```python
from build123d import *

# Parameters (mm, degrees)
BOSS_EXTRUDE1_DEPTH = 30
SKETCH2_R           = 2.25
CUT_EXTRUDE1_DEPTH  = 15
FILLET1_R           = 5
CHAMFER1_SIZE       = 20
CHAMFER1_SIZE_2     = 54.949548389
SKETCH3_W           = 25
SKETCH3_H           = 39.596952294
CUT_EXTRUDE2_DEPTH  = 15
SKETCH4_R           = 1.75
CUT_EXTRUDE3_DEPTH  = 65.75337829
CHAMFER2_SIZE       = 1
SKETCH5_R           = 2
CUT_EXTRUDE4_DEPTH  = 56.767373974
SKETCH6_R           = 7.5
CUT_EXTRUDE5_DEPTH  = 25
FILLET2_R           = 2
FILLET3_R           = 5


with BuildPart() as part:
    # Sketch1 → Boss-Extrude1 (new body)
    with BuildSketch(Plane.XY):
        with BuildLine():
            Line((-12, 0), (-12, -30))
            Line((-12, -30), (-19, -30))
            Line((-19, -30), (-19, 43))
            Line((-19, 43), (19, 43))
            Line((19, 43), (19, -30))
            Line((19, -30), (12, -30))
            Line((12, -30), (12, 0))
            ThreePointArc((12, 0), (0, 12), (-12, 0))
        make_face()
    extrude(amount=BOSS_EXTRUDE1_DEPTH)

    # Sketch2 → Cut-Extrude1 (cut)
    with BuildSketch(Plane.XZ.offset(30)):
        with Locations(Location((-15, 5, 0), (0, 0, 270))):
            Circle(SKETCH2_R)
        with Locations(Location((15, 5, 0), (0, 0, 270))):
            Circle(SKETCH2_R)
        with Locations(Location((-15, 15, 0), (0, 0, 270))):
            Circle(SKETCH2_R)
        with Locations(Location((15, 15, 0), (0, 0, 270))):
            Circle(SKETCH2_R)
        with Locations(Location((-15, 25, 0), (0, 0, 270))):
            Circle(SKETCH2_R)
        with Locations(Location((15, 25, 0), (0, 0, 270))):
            Circle(SKETCH2_R)
    extrude(amount=-CUT_EXTRUDE1_DEPTH, mode=Mode.SUBTRACT)

    # Fillet1
    fillet1_edges = [part.edges().sort_by_distance(p)[0] for p in [
        (0, 43, 0),
    ]]
    fillet(fillet1_edges, radius=FILLET1_R)

    # Chamfer1
    # the kernel refuses this chamfer: 54.949548389, 20 mm, written as the material it takes off along each edge
    with BuildSketch(Plane(origin=(-161.549828987, 43, 30), x_dir=(0, 0.09904090225205052, -0.9950833631817486), z_dir=(1, 0, 0))) as chamfer1_piece_1:
        Polygon((CHAMFER1_SIZE * 0.995083363182, -CHAMFER1_SIZE * 0.0990409022521), (-CHAMFER1_SIZE_2 * 0.0990409022522, -CHAMFER1_SIZE_2 * 0.995083363183), (0, 0), align=None)
    extrude(amount=323.099657974, mode=Mode.SUBTRACT)

    # Sketch3 → Cut-Extrude2 (cut)
    with BuildSketch(Plane(origin=(0, 43, 0), x_dir=(1, 0, 0), z_dir=(0, 1, 0))):
        Rectangle(SKETCH3_W, SKETCH3_H)
    extrude(amount=-CUT_EXTRUDE2_DEPTH, mode=Mode.SUBTRACT)

    # Sketch4 → Cut-Extrude3 (cut, through all)
    with BuildSketch(Plane.ZY.offset(19)):
        with Locations((5, 38)):
            Circle(SKETCH4_R)
    extrude(amount=-CUT_EXTRUDE3_DEPTH, mode=Mode.SUBTRACT)

    # Chamfer2
    # the kernel refuses this chamfer: 1 mm, written as the material it takes off along each edge
    with BuildSketch(Plane(origin=(-15, -30, 25), x_dir=(0, 0, -1), z_dir=(-1, 0, 0))) as chamfer2_piece_1:
        Polygon((2.25 + CHAMFER2_SIZE, 0), (2.25, -CHAMFER2_SIZE), (2.25, 0), align=None)
    revolve(axis=Axis((-15, -30, 25), (0, -1, 0)), mode=Mode.SUBTRACT)
    with BuildSketch(Plane(origin=(15, -30, 15), x_dir=(0, 0, -1), z_dir=(-1, 0, 0))) as chamfer2_piece_2:
        Polygon((2.25 + CHAMFER2_SIZE, 0), (2.25, -CHAMFER2_SIZE), (2.25, 0), align=None)
    revolve(axis=Axis((15, -30, 15), (0, -1, 0)), mode=Mode.SUBTRACT)
    with BuildSketch(Plane(origin=(-15, -30, 15), x_dir=(0, 0, -1), z_dir=(-1, 0, 0))) as chamfer2_piece_3:
        Polygon((2.25 + CHAMFER2_SIZE, 0), (2.25, -CHAMFER2_SIZE), (2.25, 0), align=None)
    revolve(axis=Axis((-15, -30, 15), (0, -1, 0)), mode=Mode.SUBTRACT)
    with BuildSketch(Plane(origin=(15, -30, 5), x_dir=(0, 0, -1), z_dir=(-1, 0, 0))) as chamfer2_piece_4:
        Polygon((2.25 + CHAMFER2_SIZE, 0), (2.25, -CHAMFER2_SIZE), (2.25, 0), align=None)
    revolve(axis=Axis((15, -30, 5), (0, -1, 0)), mode=Mode.SUBTRACT)
    with BuildSketch(Plane(origin=(15, -30, 25), x_dir=(0, 0, -1), z_dir=(-1, 0, 0))) as chamfer2_piece_5:
        Polygon((2.25 + CHAMFER2_SIZE, 0), (2.25, -CHAMFER2_SIZE), (2.25, 0), align=None)
    revolve(axis=Axis((15, -30, 25), (0, -1, 0)), mode=Mode.SUBTRACT)
    with BuildSketch(Plane(origin=(-15, -30, 5), x_dir=(0, 0, -1), z_dir=(-1, 0, 0))) as chamfer2_piece_6:
        Polygon((2.25 + CHAMFER2_SIZE, 0), (2.25, -CHAMFER2_SIZE), (2.25, 0), align=None)
    revolve(axis=Axis((-15, -30, 5), (0, -1, 0)), mode=Mode.SUBTRACT)

    # Sketch5 → Cut-Extrude4 (cut, through all)
    with BuildSketch(Plane(origin=(0, 0, 0), x_dir=(-1, 0, 0), z_dir=(0, 0, -1))):
        with Locations((0, 23)):
            Circle(SKETCH5_R)
    extrude(amount=-CUT_EXTRUDE4_DEPTH, mode=Mode.SUBTRACT)

    # Sketch6 → Cut-Extrude5 (cut)
    with BuildSketch(Plane.XY.offset(30)):
        with Locations((0, 23)):
            Circle(SKETCH6_R)
    extrude(amount=-CUT_EXTRUDE5_DEPTH, mode=Mode.SUBTRACT)

    # Fillet2
    fillet2_edges = [part.edges().sort_by_distance(p)[0] for p in [
        (-5.590169944, 28, 10.229776757),
        (5.590169944, 28, 10.229776757),
    ]]
    fillet(fillet2_edges, radius=FILLET2_R)

    # Fillet3
    fillet3_edges = [part.edges().sort_by_distance(p)[0] for p in [
        (-15.75, 43, 10),
        (15.75, 43, 10),
    ]]
    fillet(fillet3_edges, radius=FILLET3_R)


solid = part.part
```
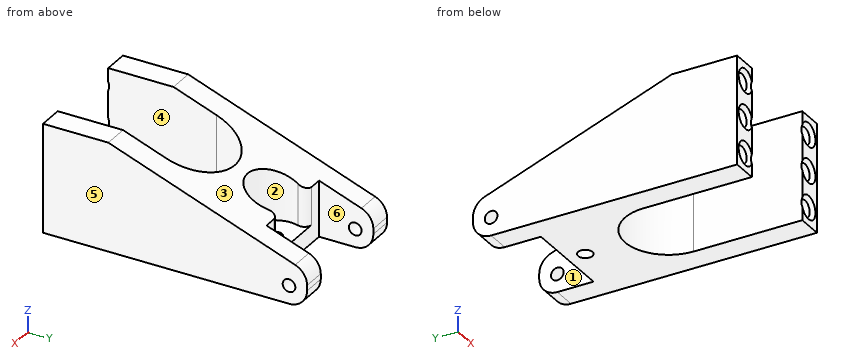
Check sheet for the modelled part. Datum: model origin and axes. Units: mm. Face numbers are marked on the shaded views. A direction names the side the tool comes from. Give positions to 0.01 mm unless a question says otherwise; leave off trailing zeros. Order: outer loops, then holes, each group sorted by start corner. A loop starts at its lowest first (then second) coordinate and runs counter-clockwise, first axis right, second up. Notation, with made-up numbers: M 7.25,-17 L 11.25,-17 A29 cw 11.25,17 Z; hole C -39.75,-30.5 d6. An arc over 180 degrees is marked long. Answer in a Markdown table with one row per item. Add a question column.
Q1. Access from +Z, -Z, +X, -X, +Y, -Y to the whole of each face (thin tool, end or side, straight path). Record for the marked faces 4, 5 and 6.
Q2. Sectioned sample at C-C, the plane y = 11. Record the boundary of the cut face in (x, z).
Q3. Sectioned sample at A-A, the plane y = -24.5. Record the boundary of the cut face in (x, z).
Q4. Sectioned sample at D-D, the plane z = 9.5. Record the boundary of the cut face in (x, y).
Q5. Release check for a two-part mould opening along Y. For the marked faces 1, 2 and 3 record: released by +Y, released by -Y, zero draft, split by the parting line, or undercut.
Q6. Thickness scan on L1, parallel to X at y = -18.5, z = 25; L2, parallel to X at y = -8, z = 8; L3, parallel to X at y = 8, z = 18.5. Record the ranges inside material, lowest first.
Q7. Gauge pin test, flat ends, axial feed: pin 1 Ø3.5 at (x, z) = (-14.5, 24) entering from -Y; pin 2 Ø4 at (x, y) = (4.5, 24.5) entering from +Z; pin 3 Ø3 at (x, z) = (0, 14) entering from -Y; pin 4 Ø3.5 at (x, y) = (0, 23) entering from +Z. Record the tip position at first contact, or that the pin passes through.
Q8. Sectioned sample at B-B, the plane x = 15. Record the boundary of the cut face in (y, z), and give its area (3 significant figures).
Verdict:
| question | item | result |
|---|---|---|
| 1 | face 4 | +Z, -Z, -Y |
| 1 | face 5 | +Z, -Z, +X, +Y, -Y |
| 1 | face 6 | +Z, -Z, +Y |
| 2 | outline | M -19,0 L -4.8,0 L -4.8,21.65 L -19,21.65 Z; M 4.8,0 L 19,0 L 19,21.65 L 4.8,21.65 Z |
| 3 | outline | M -19,0 L -12,0 L -12,30 L -19,30 Z; M 12,0 L 19,0 L 19,30 L 12,30 Z; hole C -15,5 d4.5; hole C -15,15 d4.5; hole C -15,25 d4.5; hole C 15,5 d4.5; hole C 15,15 d4.5; hole C 15,25 d4.5 |
| 4 | outline | M -19,-30 L -12,-30 L -12,0 A12 cw 12,0 L 12,-30 L 19,-30 L 19,42 L 12.5,42 L 12.5,28 L 9.01,28 A2 ccw 7.12,25.37 A7.5 cw long -7.12,25.37 A2 ccw -9.01,28 L -12.5,28 L -12.5,42 L -19,42 Z |
| 5 | face 1 | zero draft |
| 5 | face 2 | undercut |
| 5 | face 3 | released by +Y |
| 6 | L1 | -19 to -17.25, -12.75 to -12, 12 to 12.75, 17.25 to 19 |
| 6 | L2 | -19 to -12, 12 to 19 |
| 6 | L3 | -19 to -8.94, 8.94 to 19 |
| 7 | pin 1 | y = -29.62 |
| 7 | pin 2 | z = 5 |
| 7 | pin 3 | y = 11.91 |
| 7 | pin 4 | through |
| 8 | outline | M -30,0 L 38,0 A5 ccw 43,5 L 43,6.5 A5 ccw 39.71,11.2 L -11.95,30 L -30,30 L -30,28.25 L -29,27.25 L -15,27.25 L -15,22.75 L -29,22.75 L -30,21.75 L -30,18.25 L -29,17.25 L -15,17.25 L -15,12.75 L -29,12.75 L -30,11.75 L -30,8.25 L -29,7.25 L -15,7.25 L -15,2.75 L -29,2.75 L -30,1.75 Z; hole C 38,5 d3.5 |
| 8 | area | 1,420 mm² |
